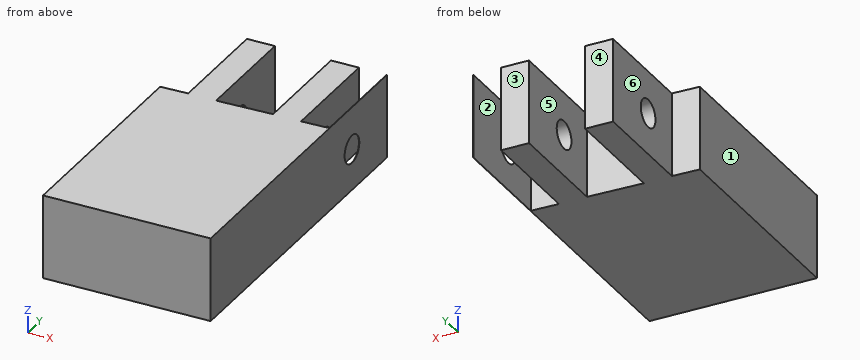
```python
from build123d import *

# Parameters (mm, degrees)
F0_W     = 76.2
F0_H     = 38.1
F1_DEPTH = 76.2
F3_R     = 6.35
F4_DEPTH = 85.344
F6_DEPTH = 50.8


with BuildPart() as f1:
    # F0 (on Front) → F1 (new body, symmetric)
    with BuildSketch(Plane.XZ):
        with Locations((-179.678692, 19.05)):
            Rectangle(F0_W, F0_H)
    extrude(amount=F1_DEPTH, both=True)


with BuildPart() as f1_1:
    # F2: moved
    add(f1.part.moved(Location((141.732, 0, -12.446))))

    # F3 (on Right) → F4 (cut, symmetric)
    with BuildSketch(Plane.YZ):
        with Locations((45.916668, 6.35)):
            Circle(F3_R)
    extrude(amount=F4_DEPTH, both=True, mode=Mode.SUBTRACT)

    # F5 (on Top) → F6 (cut, symmetric)
    with BuildSketch(Plane.XY):
        Polygon((-63.508823, 25.400016), (-63.508823, 76.200016), (-76.920537, 76.956743), (-76.920537, 25.001949), align=None)
        Polygon((-25.313061, 76.956743), (-50.808823, 76.200016), (-50.808823, 25.400016), (-25.313061, 26.156743), align=None)
        Polygon((0, 76.200016), (-12.613061, 76.956743), (-12.613061, 26.156743), (0, 26.531105), align=None)
    extrude(amount=F6_DEPTH, both=True, mode=Mode.SUBTRACT)


solid = f1_1.part
```
Input: part model. Units: mm. Frame: model coordinates. Face numbers are marked on the shaded views. A direction names the side the tool comes from. Give positions to 0.01 mm unless a question says otherwise; leave off trailing zeros. Order: outer loops, then holes, each group sorted by start corner. A loop starts at its lowest first (then second) coordinate and runs counter-clockwise, first axis right, second up. Notation, with made-up numbers: (-25.75, 16.5) - (-9.75, 16.5) arc R16 ccw to (-9.75, 35.5) - close; hole circle Ø2 at (33, 64.25). An arc over 180 degrees is marked (long way). Use a Markdown table: item, result.
(1) Line query: line 1 (X direction, y = 31.5, z = 23.5); line 2 (Y direction, x = -59, z = 6); line 3 (Y direction, x = -54.5, z = 12). Output: solid intervals per line, ascending. Write a range as from..to.
Computed values:
| item | result |
|---|---|
| line 1 | x = -63.51..-50.81, -25.31..-12.61, 0..0.15 |
| line 2 | y = -76.2..39.58, 52.26..76.2 |
| line 3 | y = -76.2..43.02, 48.81..76.2 |
(2) Section query B-B (y = 49). Output: boundary loops of the cut face in (x, z).
Computed values:
| item | result |
|---|---|
| outline | (-63.51, -12.45) - (-50.81, -12.45) - (-50.81, 0.8) - (-63.51, 0.8) - close; (-63.51, 11.9) - (-50.81, 11.9) - (-50.81, 25.65) - (-63.51, 25.65) - close; (-25.31, -12.45) - (-12.61, -12.45) - (-12.61, 0.8) - (-25.31, 0.8) - close; (-25.31, 11.9) - (-12.61, 11.9) - (-12.61, 25.65) - (-25.31, 25.65) - close; (0, -12.45) - (0.15, -12.45) - (0.15, 0.8) - (0, 0.8) - close; (0, 11.9) - (0.15, 11.9) - (0.15, 25.65) - (0, 25.65) - close |
(3) Section query A-A (z = 6.35). Output: boundary loops of the cut face in (x, y).
Computed values:
| item | result |
|---|---|
| outline | (-76.05, -76.2) - (0.15, -76.2) - (0.15, 39.57) - (0, 39.57) - (0, 26.53) - (-12.61, 26.16) - (-12.61, 39.57) - (-25.31, 39.57) - (-25.31, 26.16) - (-50.81, 25.4) - (-50.81, 39.57) - (-63.51, 39.57) - (-63.51, 25.4) - (-76.05, 25.03) - close; (-63.51, 52.27) - (-50.81, 52.27) - (-50.81, 76.2) - (-63.51, 76.2) - close; (-25.31, 52.27) - (-12.61, 52.27) - (-12.61, 76.2) - (-25.31, 76.2) - close; (0, 52.27) - (0.15, 52.27) - (0.15, 76.2) - (0, 76.2) - close |
(4) Access query for the marked faces 4, 5 and 6. Directions: +Z, -Z, +X, -X, +Y, -Y. A direction counts if a zero-diameter tool reaches every point of the face in a straight line with its end or side. Return the directions, or none.
Computed values:
| item | result |
|---|---|
| face 4 | +Z, -Z, +X, -X, +Y |
| face 5 | +Z, -Z, +Y |
| face 6 | +Z, -Z, -X, +Y |
(5) Section query C-C (z = -8.5). Output: boundary loops of the cut face in (x, y).
Computed values:
| item | result |
|---|---|
| outline | (-76.05, -76.2) - (0.15, -76.2) - (0.15, 76.2) - (0, 76.2) - (0, 26.53) - (-12.61, 26.16) - (-12.61, 76.2) - (-25.31, 76.2) - (-25.31, 26.16) - (-50.81, 25.4) - (-50.81, 76.2) - (-63.51, 76.2) - (-63.51, 25.4) - (-76.05, 25.03) - close |
(6) Draft query along X for the marked faces 1, 2 and 3. Return one class per face: released by +X, released by -X, zero draft, split by the parting line, or undercut.
Computed values:
| item | result |
|---|---|
| face 1 | released by -X |
| face 2 | undercut |
| face 3 | zero draft |
(7) Pin query (flat end, axial travel): pin 1 (11.5 mm diameter, centred on y = 47.5, z = -2.5, fed in from -X). Return the tip coordinate at first contact, or that it passes through.
Computed values:
| item | result |
|---|---|
| pin 1 | stops at x = -63.51 |
